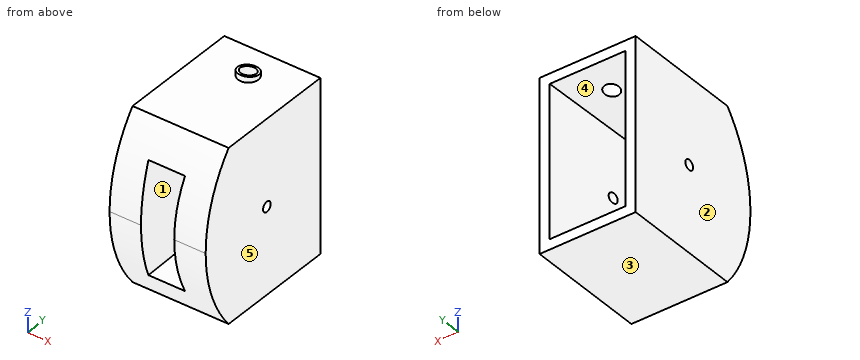
from build123d import *

# Parameters (mm, degrees)
SKETCH1_W                    = 190
SKETCH1_H                    = 340
BOSS_EXTRUDE1_DEPTH          = 300
SKETCH2_R                    = 20
SKETCH2_R_2                  = 15
BOSS_EXTRUDE2_DEPTH          = 57
CUT_EXTRUDE1_START           = -190
SKETCH5_R                    = 10
CUT_EXTRUDE1_DEPTH           = 612.460555687
CUT_EXTRUDE2_DEPTH           = 422.460555687
CUT_EXTRUDE6_START           = -236
CUT_EXTRUDE6_DEPTH           = 236
SKETCH10_OUTSIDE_W           = 383.134
SKETCH10_OUTSIDE_H           = 590.134
SKETCH10_OUTSIDE_W_2         = 190
SKETCH10_OUTSIDE_H_2         = 340
CUT_EXTRUDE7_DEPTH           = 301
CUT_EXTRUDE7_DRAFT           = -8
SKETCH10_OUTSIDE_W_3         = 150
SKETCH10_OUTSIDE_H_3         = 300
CUT_EXTRUDE7_PROFILE_2_DEPTH = 301
CUT_EXTRUDE7_PROFILE_2_DRAFT = -8


with BuildPart() as part:
    # Sketch1 → Boss-Extrude1 (new body)
    with BuildSketch(Plane(origin=(0, 0, 0), x_dir=(1, 0, 0), z_dir=(0, 1, 0))):
        Rectangle(SKETCH1_W, SKETCH1_H)
    extrude(amount=BOSS_EXTRUDE1_DEPTH)

    # Sketch2 → Boss-Extrude2 (add)
    with BuildSketch(Plane.XY.offset(170)):
        with Locations(Location((0, 237, 0), (0, 0, 180))):
            Circle(SKETCH2_R)
        with Locations(Location((0, 237, 0), (0, 0, 180))):
            Circle(SKETCH2_R_2, mode=Mode.SUBTRACT)
    extrude(amount=BOSS_EXTRUDE2_DEPTH)

    # Sketch5 → Cut-Extrude1 (cut, through all)
    with BuildSketch(Plane.ZY.offset(95).offset(CUT_EXTRUDE1_START)):
        with Locations((0, 160)):
            Circle(SKETCH5_R)
    extrude(amount=CUT_EXTRUDE1_DEPTH, mode=Mode.SUBTRACT)

    # Sketch9 → Cut-Extrude2 (cut, through all)
    with BuildSketch(Plane.ZY.offset(95)):
        with BuildLine():
            ThreePointArc((0, 0), (-90.138848958, 15.439927953), (-170, 60))
            Line((-170, 60), (-170, 0))
            Line((-170, 0), (0, 0))
        make_face()
        with BuildLine():
            ThreePointArc((170, 60), (90.138848958, 15.439927953), (0, 0))
            Line((0, 0), (170, 0))
            Line((170, 0), (170, 60))
        make_face()
    extrude(amount=-CUT_EXTRUDE2_DEPTH, mode=Mode.SUBTRACT)

    # Sketch2<3> → Cut-Extrude6 (cut)
    with BuildSketch(Plane.XY.offset(170).offset(CUT_EXTRUDE6_START)):
        with BuildLine():
            ThreePointArc((-15, 237), (0, 222), (15, 237))
            Line((15, 237), (-15, 237))
        make_face()
        with BuildLine():
            Line((-15, 237), (15, 237))
            ThreePointArc((15, 237), (0, 252), (-15, 237))
        make_face()
    extrude(amount=CUT_EXTRUDE6_DEPTH, mode=Mode.SUBTRACT)


with BuildPart() as cut_extrude7_tool:
    # Sketch10 outside → Cut-Extrude7 (with draft: the straight prism first)
    with BuildSketch(Plane(origin=(0, 300, 0), x_dir=(1, 0, 0), z_dir=(0, 1, 0))):
        with Locations((0, -28.5)):
            Rectangle(SKETCH10_OUTSIDE_W, SKETCH10_OUTSIDE_H)
        Rectangle(SKETCH10_OUTSIDE_W_2, SKETCH10_OUTSIDE_H_2, mode=Mode.SUBTRACT)
    extrude(amount=-CUT_EXTRUDE7_DEPTH)
    # Cut-Extrude7: the draft: its side faces are tilted about the plane it starts from
    cut_extrude7_sides = [cut_extrude7_tool.faces().sort_by_distance(p)[0] for p in [
        (0, 149.5, 323.567),
        (191.567, 149.5, 28.5),
        (0, 149.5, -266.567),
        (-191.567, 149.5, 28.5),
        (0, 149.5, -170),
        (95, 149.5, 0),
        (0, 149.5, 170),
        (-95, 149.5, 0),
    ]]
    draft(cut_extrude7_sides, Plane(origin=(0, 300, 0), x_dir=(1, 0, 0), z_dir=(0, 1, 0)), CUT_EXTRUDE7_DRAFT)


with BuildPart() as part_1:
    add(part.part)

    # Cut-Extrude7: cut by cut_extrude7_tool
    add(cut_extrude7_tool.part, mode=Mode.SUBTRACT)


with BuildPart() as cut_extrude7_profile_2_tool:
    # Sketch10 outside → Cut-Extrude7 profile 2 (with draft: the straight prism first)
    with BuildSketch(Plane(origin=(0, 300, 0), x_dir=(1, 0, 0), z_dir=(0, 1, 0))):
        Rectangle(SKETCH10_OUTSIDE_W_3, SKETCH10_OUTSIDE_H_3)
    extrude(amount=-CUT_EXTRUDE7_PROFILE_2_DEPTH)
    # Cut-Extrude7 profile 2: the draft: its side faces are tilted about the plane it starts from
    cut_extrude7_profile_2_sides = [cut_extrude7_profile_2_tool.faces().sort_by_distance(p)[0] for p in [
        (-75, 149.5, 0),
        (0, 149.5, 150),
        (75, 149.5, 0),
        (0, 149.5, -150),
    ]]
    draft(cut_extrude7_profile_2_sides, Plane(origin=(0, 300, 0), x_dir=(1, 0, 0), z_dir=(0, 1, 0)), CUT_EXTRUDE7_PROFILE_2_DRAFT)


with BuildPart() as part_2:
    add(part_1.part)

    # Cut-Extrude7 profile 2: cut by cut_extrude7_profile_2_tool
    add(cut_extrude7_profile_2_tool.part, mode=Mode.SUBTRACT)


solid = part_2.part
Read the model definition and answer for the solid it produces. Units are mm, in the model's axes. Face numbers are marked on the shaded views. A direction names the side the tool comes from. Round coordinates to 2 decimals unless told otherwise and drop trailing zeros. Write each loop counter-clockwise with the first axis right and the second up, starting at its lowest first coordinate (ties: lowest second). Pieces come first, ordered by that corner, then holes.
Q1. The mould has two halves that part along X. Classify the marked faces 1, 2 and 3: released by +X, released by -X, zero draft, split by the parting line, or undercut.
Values:
face 1: undercut
face 2: released by -X
face 3: zero draft
Q2. Find section D-D on x = 60. Determine the outline of the cut face in (y, z), and give its area (3 significant figures).
Values:
outline: (0, 0) arc R270.83 ccw to (60, -170) - (300, -170) - (300, -150) - (193.27, -135) - (193.27, 135) - (300, 150) - (300, 170) - (60, 170) arc R270.83 ccw to start; hole circle Ø20 at (160, 0)
area: 64,800 mm2
Q3. Find section C-C on y = 160. Determine the outline of the cut face in (x, z).
Values:
outline: (-95, -170) - (95, -170) - (95, -10) - (55.32, -10) - (55.32, -130.32) - (-55.32, -130.32) - (-55.32, -10) - (-95, -10) - close; (-95, 10) - (-55.32, 10) - (-55.32, 130.32) - (55.32, 130.32) - (55.32, 10) - (95, 10) - (95, 170) - (-95, 170) - close
Q4. Straight lines are drawn through the part: line 1 (Z direction, x = 77, y = 160); line 2 (X direction, y = 150, z = 122.5); line 3 (Y direction, x = 0, z = 162). For each, find the intervals that lie inside material, in ascending order.
Values:
line 1: z = -170 to -10, 10 to 170
line 2: x = -95 to -53.92, 53.92 to 95
line 3: y = 53.79 to 222, 252 to 300
Q5. Find section A-A on z = -91. Determine the outline of the cut face in (x, y).
Values:
outline: (-95, 15.75) - (-35.05, 15.75) - (-75, 300) - (-95, 300) - close; (35.05, 15.75) - (95, 15.75) - (95, 300) - (75, 300) - close
Q6. A tool of negligible diameter and unlimited length cuts with its end or side. For the marked faces 4 and 5, from which of +Z, -Z, +X, -X, +Y, -Y can it reach the whole face along a straight path? Write none if from no direction.
Values:
face 4: +Y
face 5: +Z, -Z, +X, +Y, -Y
Q7. Flat-ended cylindrical pins translate along their axes: P1, Ø1.5, axis at x = 44.5, z = -77, coming from the -Y side (3 decimals); P2, Ø3, axis at x = -76, z = -117.5, coming from the -Y side; P3, Ø10, axis at x = 37.5, y = 51.5, coming from the -Z side. Find the tip coordinate at first contact, or state that the pin passes through.
Values:
P1: stops at y = 10.955
P2: stops at y = 26.1
P3: stops at z = -165.57
